Part print with two shaded views. Sizes in mm from the minimum x, y, z corner. Give positions to 0.01 mm unless a question says otherwise; leave off trailing zeros. Order: outer loops, then holes, each group sorted by start corner. A loop starts at its lowest first (then second) coordinate and runs counter-clockwise, first axis right, second up. Notation, with made-up numbers: (-7.5, -14) - (1.5, -14) arc R12 cw to (1.5, -2) - close; hole circle Ø10 at (69.25, -22). An arc over 180 degrees is marked (long way). Return JSON: item names as keys, results as strings. Group by question number.
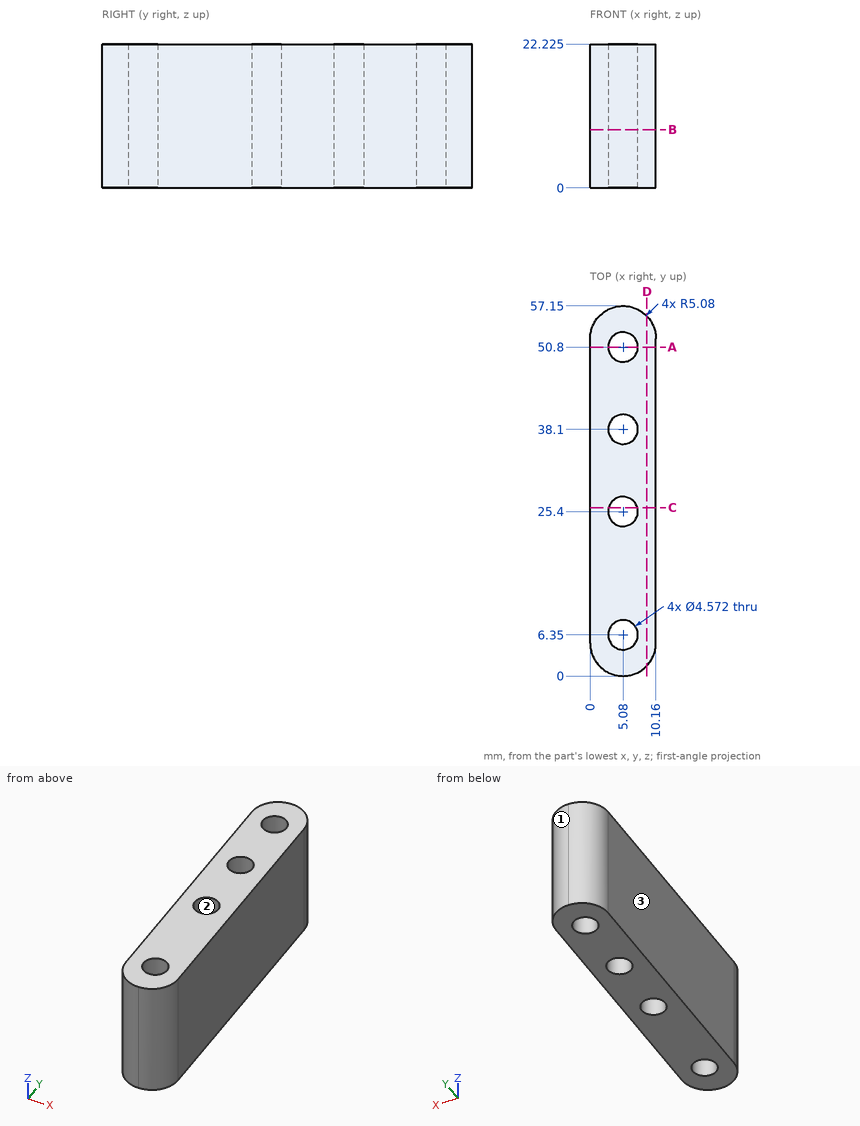
(1) Drill centre lines: L1, parallel to Y at x = 5.08, z = 16.25; L2, parallel to Y at x = 4, z = 11 (1 decimal); L3, parallel to X at y = 38.5, z = 4.25. Where is each one in solid material? Low to high.
(2) Pull direction X, two halves, no side cores. Call the marked faces 1, 2 and 3: released by +X, released by -X, zero draft, split by the parting line, or undercut.
(3) Slice it at D-D (x = 8.75). Give the cut face in (y, z) (1 decimal), and give its area (3 significant figures).
(4) Slice it at B-B (z = 9). State how many separate pieces and enclosed holes the cut face has, and give its area (3 significant figures).
(5) Slice it at A-A (y = 50.8). Give the cut face in (x, z) (3 decimals), and give its area (3 significant figures).
(6) Slice it at C-C (y = 26). Give the cut face in (x, z) (3 decimals), and give its area (3 significant figures).
Result set:
{
 "1": {"L1": "y = 0 to 4.06, 8.64 to 23.11, 27.69 to 35.81, 40.39 to 48.51, 53.09 to 57.15", "L2": "y = 0.1 to 4.3, 8.4 to 23.4, 27.4 to 36.1, 40.1 to 48.8, 52.8 to 57", "L3": "x = 0 to 2.83, 7.33 to 10.16"},
 "2": {"face 1": "released by +X", "face 2": "undercut", "face 3": "released by -X"},
 "3": {"outline": "(1.6, 0) - (55.6, 0) - (55.6, 22.2) - (1.6, 22.2) - close", "area": "1,200 mm²"},
 "4": {"separate pieces": "1", "enclosed holes": "4", "area": "493 mm²"},
 "5": {"outline": "(0, 0) - (2.794, 0) - (2.794, 22.225) - (0, 22.225) - close; (7.366, 0) - (10.16, 0) - (10.16, 22.225) - (7.366, 22.225) - close", "area": "124 mm²"},
 "6": {"outline": "(0, 0) - (2.874, 0) - (2.874, 22.225) - (0, 22.225) - close; (7.286, 0) - (10.16, 0) - (10.16, 22.225) - (7.286, 22.225) - close", "area": "128 mm²"}
}
